Build history of the part. All positions in model axes, mm. A direction names the side the tool comes from. Give positions to 0.01 mm unless a question says otherwise; leave off trailing zeros. Order: outer loops, then holes, each group sorted by start corner. A loop starts at its lowest first (then second) coordinate and runs counter-clockwise, first axis right, second up. Notation, with made-up numbers: (39.5, 77) -> (90.5, 77) arc R7 cw to (90.5, 87) -> close; hole circle Ø4 at (3, 0.25). An arc over 180 degrees is marked (long way). One line per question, with ' | ' between items. Start each with the question number.
(1) Cut at D-D (z = 41). Give the cut face in (x, y), then the cut area to 3 significant figures.
(2) Cut at B-B (y = 3.25). Give the cut face in (x, z), then the cut area to 3 significant figures.
(3) Drill centre lines: L1, parallel to X at y = 5.1, z = 37.5; L2, parallel to Z at x = 0, y = 6.4; L3, parallel to Z at x = 0, y = 2. Where is each one in solid material? Low to high. Write a range as from..to.
(4) Pull direction Y, two halves, no side cores. Call faces 1 (the face through (0, 3, -26.133)), 2 (the face through (-0.414, 3.458, 49.493)), 3 (the face through (0, 0, -4)): +Y half, -Y half, draft (parallel to the pull), parting line (faces both ways), or undercut.
(5) Cut at A-A (z = -37.5). Give the cut face in (x, y), then the cut area to 3 significant figures.
(6) Pin check, flat tips, straight feed: pin 1 Ø3 at (y, z) = (2.5, -12) entering from +X; pin 2 Ø2 at (x, y) = (8, 1) entering from +Z; pin 3 Ø1.5 at (x, y) = (-1, 3) entering from -Z. Stop position of each tip, or through.
(7) Cut at C-C (x = 0). Give the cut face in (y, z).
(8) Which spindle directions (+Z, -Z, +X, -X, +Y, -Y) get a long thin tool onto all of the face, cutting with end or side? Do faces 4 (the face through (2.7, 0.5, 27.7)), 5 (the face through (2.7, 6.5, 27.7)), 6 (the face through (-7, 1, -45)), 7 (the face through (7.5, 3, 0)). Say none if no direction does.
from build123d import *

# Parameters (mm, degrees)
PROFILE_SKETCH_R                  = 10
PROFILE_EXTRUDE_DEPTH             = 7
UPPER_WRIST_CUT_DEPTH             = 0.5
LOWER_START                       = 6.5
LOWER_WRIST_CUT_DEPTH             = 0.5
FINGER_CUT_REACH                  = 53.413
FINGER_CUT_END_RADIUS             = 12
FINGER_CUT_SKETCH_W               = 23.367496998
FINGER_CUT_SKETCH_H               = 5
FINGER_CUT_DIRECTION_2_REACH      = 53.413
FINGER_CUT_DIRECTION_2_END_RADIUS = 12


with BuildPart() as part:
    # Profile Sketch → Profile Extrude (new body)
    with BuildSketch(Plane(origin=(0, 0, 0), x_dir=(1, 0, 0), z_dir=(0, 1, 0))):
        with BuildLine():
            Line((-7.5, 28.132503002), (-7.5, -28.132503002))
            ThreePointArc((-7.5, -28.132503002), (0, -49.5), (7.5, -28.132503002))
            Line((7.5, -28.132503002), (7.5, 28.132503002))
            ThreePointArc((7.5, 28.132503002), (0, 49.5), (-7.5, 28.132503002))
        make_face()
        with Locations(Location((0, -37.5, 0), (0, 0, 270))):
            Circle(PROFILE_SKETCH_R, mode=Mode.SUBTRACT)
        with Locations(Location((0, 37.5, 0), (0, 0, 270))):
            Circle(PROFILE_SKETCH_R, mode=Mode.SUBTRACT)
    extrude(amount=PROFILE_EXTRUDE_DEPTH)

    # Wrist Cut Sketch → Upper Wrist Cut (cut)
    with BuildSketch(Plane(origin=(0, 0, 0), x_dir=(1, 0, 0), z_dir=(0, 1, 0))):
        with BuildLine():
            Line((-7.5, -28.132503002), (-7.5, -25.5))
            Line((-7.5, -25.5), (7.5, -25.5))
            Line((7.5, -25.5), (7.5, -28.132503002))
            ThreePointArc((7.5, -28.132503002), (0, -49.5), (-7.5, -28.132503002))
        make_face()
    extrude(amount=UPPER_WRIST_CUT_DEPTH, mode=Mode.SUBTRACT)

    # Sketch2<2> → Lower Wrist Cut (cut)
    with BuildSketch(Plane(origin=(0, 0, 0), x_dir=(1, 0, 0), z_dir=(0, 1, 0)).offset(LOWER_START)):
        with BuildLine():
            Line((-7.5, -28.132503002), (-7.5, -25.5))
            Line((-7.5, -25.5), (7.5, -25.5))
            Line((7.5, -25.5), (7.5, -28.132503002))
            ThreePointArc((7.5, -28.132503002), (0, -49.5), (-7.5, -28.132503002))
        make_face()
    extrude(amount=LOWER_WRIST_CUT_DEPTH, mode=Mode.SUBTRACT)

    # Finger Cut: up to this cylinder (the profile starts inside it)
    finger_cut_end = Plane(origin=(0, 3.5, -37.5), z_dir=(0, -1, 0)) * Cylinder(FINGER_CUT_END_RADIUS, 131.826, mode=Mode.PRIVATE)
    # Finger Cut Sketch → Finger Cut (cut, up to the surface)
    with BuildSketch(Plane(origin=(0, 0, 0), x_dir=(0, 0, -1), z_dir=(1, 0, 0)), mode=Mode.PRIVATE) as finger_cut_sk1:
        with Locations((37.816251501, 3.5)):
            Rectangle(FINGER_CUT_SKETCH_W, FINGER_CUT_SKETCH_H)
    finger_cut_tool1 = extrude(finger_cut_sk1.sketch, amount=-FINGER_CUT_REACH, mode=Mode.PRIVATE) & finger_cut_end
    add(finger_cut_tool1.solids().sort_by_distance((0, 3.5, -37.816252))[0], mode=Mode.SUBTRACT)

    # Finger Cut direction 2: up to this cylinder (the profile starts inside it)
    finger_cut_direction_2_end = Plane(origin=(0, 3.5, -37.5), z_dir=(0, -1, 0)) * Cylinder(FINGER_CUT_DIRECTION_2_END_RADIUS, 131.826, mode=Mode.PRIVATE)
    # Finger Cut Sketch → Finger Cut direction 2 (cut, up to the surface)
    with BuildSketch(Plane(origin=(0, 0, 0), x_dir=(0, 0, -1), z_dir=(1, 0, 0)), mode=Mode.PRIVATE) as finger_cut_direction_2_sk1:
        with Locations((37.816251501, 3.5)):
            Rectangle(FINGER_CUT_SKETCH_W, FINGER_CUT_SKETCH_H)
    finger_cut_direction_2_tool1 = extrude(finger_cut_direction_2_sk1.sketch, amount=FINGER_CUT_DIRECTION_2_REACH, mode=Mode.PRIVATE) & finger_cut_direction_2_end
    add(finger_cut_direction_2_tool1.solids().sort_by_distance((0, 3.5, -37.816252))[0], mode=Mode.SUBTRACT)


solid = part.part
Result set:
1) outline: (-11.48, 0.5) -> (-9.37, 0.5) -> (-9.37, 6.5) -> (-11.48, 6.5) -> close; (9.37, 0.5) -> (11.48, 0.5) -> (11.48, 6.5) -> (9.37, 6.5) -> close | area: 25.3 mm2
2) outline: (-7.5, -28.13) arc R12 cw to (-3.84, -26.13) -> (3.84, -26.13) arc R12 cw to (7.5, -28.13) -> (7.5, 28.13) arc R12 ccw (long way) to (-7.5, 28.13) -> close; hole circle Ø20 at (0, 37.5) | area: 932 mm2
3) L1: x = -12..-10, 10..12 | L2: z = -49.5..-47.5, -27.5..27.5, 47.5..49.5 | L3: z = -26.13..27.5, 47.5..49.5
4) face 1: undercut | face 2: draft | face 3: -Y half
5) outline: (-12, 0) -> (-10, 0) -> (-10, 1) -> (-12, 1) -> close; (-12, 6) -> (-10, 6) -> (-10, 7) -> (-12, 7) -> close; (10, 0) -> (12, 0) -> (12, 1) -> (10, 1) -> close; (10, 6) -> (12, 6) -> (12, 7) -> (10, 7) -> close | area: 8.00 mm2
6) pin 1: stops at x = 7.5 | pin 2: stops at z = 47.25 | pin 3: stops at z = -26.13
7) outline: (0, -49.5) -> (1, -49.5) -> (1, -47.5) -> (0, -47.5) -> close; (0, -27.5) -> (1, -27.5) -> (1, -26.13) -> (6, -26.13) -> (6, -27.5) -> (7, -27.5) -> (7, 25.5) -> (6.5, 25.5) -> (6.5, 27.5) -> (0.5, 27.5) -> (0.5, 25.5) -> (0, 25.5) -> close; (0.5, 47.5) -> (6.5, 47.5) -> (6.5, 49.5) -> (0.5, 49.5) -> close; (6, -49.5) -> (7, -49.5) -> (7, -47.5) -> (6, -47.5) -> close
8) face 4: +Z, +X, -X, -Y | face 5: +Z, +X, -X, +Y | face 6: -Z | face 7: +X, +Y, -Y
